```python
from build123d import *

# Parameters (mm, degrees)
ESQUISSE1_W                                       = 30
ESQUISSE1_H                                       = 44.6
BOSS_EXTRU_1_DEPTH                                = 12.2
ESQUISSE2_W                                       = 30
ESQUISSE2_H                                       = 4.3
ENL_V_MAT_EXTRU_1_DEPTH                           = 17.8
ESQUISSE3_W                                       = 30
ESQUISSE3_H                                       = 4.3
ENL_V_MAT_EXTRU_2_DEPTH                           = 22.8
FRAISAGE_POUR_VIS_T_TE_FRAIS_E_BOMB_E_D           = 5.09999996
FRAISAGE_POUR_VIS_T_TE_FRAIS_E_BOMB_E_CSINK_D     = 10.500000082
FRAISAGE_POUR_VIS_T_TE_FRAIS_E_BOMB_E_CSINK_ANGLE = 90
ESQUISSE6_W                                       = 30
ESQUISSE6_H                                       = 12.2
BOSS_EXTRU_2_DEPTH                                = 26
ESQUISSE7_W                                       = 26
ESQUISSE7_H                                       = 4.3
ENL_V_MAT_EXTRU_3_DEPTH                           = 31
FRAISAGE_POUR_VIS_T_TE_FRAIS_E_BOM_2_D            = 5.09999996
FRAISAGE_POUR_VIS_T_TE_FRAIS_E_BOM_2_CSINK_D      = 10.500000082
FRAISAGE_POUR_VIS_T_TE_FRAIS_E_BOM_2_CSINK_ANGLE  = 90


with BuildPart() as part:
    # Esquisse1 → Boss.-Extru.1 (new body)
    with BuildSketch(Plane.XY):
        with Locations((-26.085427136, 14.986432161)):
            Rectangle(ESQUISSE1_W, ESQUISSE1_H)
    extrude(amount=BOSS_EXTRU_1_DEPTH)

    # Esquisse2 → Enlèv. mat.-Extru.1 (cut)
    with BuildSketch(Plane(origin=(0, 37.286432161, 0), x_dir=(1, 0, 0), z_dir=(0, 1, 0))):
        with Locations((-26.085427136, -6.1)):
            Rectangle(ESQUISSE2_W, ESQUISSE2_H)
    extrude(amount=-ENL_V_MAT_EXTRU_1_DEPTH, mode=Mode.SUBTRACT)

    # Esquisse3 → Enlèv. mat.-Extru.2 (cut)
    with BuildSketch(Plane.XZ.offset(7.313567839)):
        with Locations((-26.085427136, 6.1)):
            Rectangle(ESQUISSE3_W, ESQUISSE3_H)
    extrude(amount=-ENL_V_MAT_EXTRU_2_DEPTH, mode=Mode.SUBTRACT)

    # Fraisage pour vis _ t_te frais_e bomb_e (through all)
    with Locations(Plane(origin=(-26.085427136, -1.313567839, 12.2), x_dir=(1, 0, 0), z_dir=(0, 0, 1))):
        with Locations((0, 0), (0, 32.6)):
            CounterSinkHole(FRAISAGE_POUR_VIS_T_TE_FRAIS_E_BOMB_E_D / 2, FRAISAGE_POUR_VIS_T_TE_FRAIS_E_BOMB_E_CSINK_D / 2, counter_sink_angle=FRAISAGE_POUR_VIS_T_TE_FRAIS_E_BOMB_E_CSINK_ANGLE)

    # Esquisse6 → Boss.-Extru.2 (add)
    with BuildSketch(Plane(origin=(0, 0, 0), x_dir=(-1, 0, 0), z_dir=(0, 0, -1))):
        with Locations((26.085427136, 13.386432161)):
            Rectangle(ESQUISSE6_W, ESQUISSE6_H)
    extrude(amount=BOSS_EXTRU_2_DEPTH)

    # Esquisse7 → Enlèv. mat.-Extru.3 (cut, through all)
    with BuildSketch(Plane.ZY.offset(41.085427136)):
        with Locations((-13, 13.386432161)):
            Rectangle(ESQUISSE7_W, ESQUISSE7_H)
    extrude(amount=-ENL_V_MAT_EXTRU_3_DEPTH, mode=Mode.SUBTRACT)

    # Fraisage pour vis _ t_te frais_e bom 2 (through all)
    with Locations(Plane(origin=(-26.085427136, 7.286432161, -13), x_dir=(-1, 0, 0), z_dir=(0, -1, 0))):
        with Locations((0, 0)):
            CounterSinkHole(FRAISAGE_POUR_VIS_T_TE_FRAIS_E_BOM_2_D / 2, FRAISAGE_POUR_VIS_T_TE_FRAIS_E_BOM_2_CSINK_D / 2, counter_sink_angle=FRAISAGE_POUR_VIS_T_TE_FRAIS_E_BOM_2_CSINK_ANGLE)


solid = part.part
```
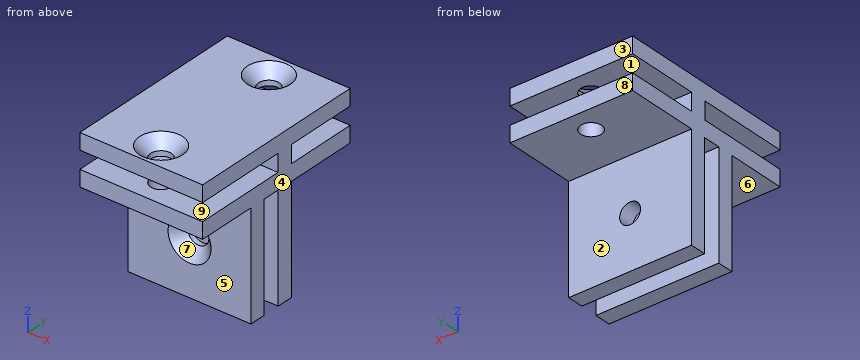
For this review, take the finished solid that the model builds, in its own axes (mm). Face numbers are marked on the shaded views. A direction names the side the tool comes from. Round coordinates to 2 decimals unless told otherwise and drop trailing zeros. Loops run counter-clockwise (first coordinate to the right, second up) from the corner with the lowest first, then second, coordinate; pieces in that order, holes last.
Q1. Insertion check: pin 1 Ø8 at (x, y) = (-26.09, 31.29) entering from +Z; pin 2 Ø5.5 at (x, y) = (-24.5, 32) entering from +Z; pin 3 Ø1.3 at (x, y) = (-29.5, 14) entering from -Z. Each pin has a flat end and moves straight along its axis. Give the tip position at first contact, or say it passes through.
Result sheet:
pin 1: stops at z = 10.96
pin 2: stops at z = 11.44
pin 3: stops at z = 0
Q2. Mouldability with a two-part tool opening along Z and no side actions: class the marked faces 6, 7, 8 and 9 as +Z half, -Z half, draft (parallel to the pull), parting line (faces both ways), or undercut.
Result sheet:
face 6: -Z half
face 7: undercut
face 8: draft
face 9: undercut
Q3. Machinability: for the marked faces 1, 2, 3, 4 and 5, which of the approach directions +Z, -Z, +X, -X, +Y, -Y give a long, thin tool a straight path to every point of the face, cutting with its end or side? Answer none if there is none.
Result sheet:
face 1: +X, -X, +Y
face 2: -Z, +X, -X, +Y
face 3: +Z, -Z, +X, -X, +Y
face 4: +Z, -Z, +X, +Y, -Y
face 5: -Z, +X, -X, -Y
Q4. Add section D-D on z = -20. Write out the cut boundary in (x, y).
Result sheet:
outline: (-41.09, 7.29) - (-11.09, 7.29) - (-11.09, 11.24) - (-41.09, 11.24) - close; (-41.09, 15.54) - (-11.09, 15.54) - (-11.09, 19.49) - (-41.09, 19.49) - close
Q5. Add section C-C on x = -38. Write out the cut boundary in (y, z), plus the area to 3 significant figures.
Result sheet:
outline: (-7.31, 0) - (7.29, 0) - (7.29, -26) - (11.24, -26) - (11.24, 0) - (15.54, 0) - (15.54, -26) - (19.49, -26) - (19.49, 0) - (37.29, 0) - (37.29, 3.95) - (19.49, 3.95) - (19.49, 8.25) - (37.29, 8.25) - (37.29, 12.2) - (-7.31, 12.2) - (-7.31, 8.25) - (15.49, 8.25) - (15.49, 3.95) - (-7.31, 3.95) - close
area: 575 mm2
Q6. Add section B-B on z = -13. Write out the cut boundary in (x, y), plus the area to 3 significant figures.
Result sheet:
outline: (-41.09, 7.29) - (-31.34, 7.29) - (-28.64, 9.99) - (-28.64, 11.24) - (-41.09, 11.24) - close; (-41.09, 15.54) - (-28.64, 15.54) - (-28.64, 19.49) - (-41.09, 19.49) - close; (-23.54, 9.99) - (-20.84, 7.29) - (-11.09, 7.29) - (-11.09, 11.24) - (-23.54, 11.24) - close; (-23.54, 15.54) - (-11.09, 15.54) - (-11.09, 19.49) - (-23.54, 19.49) - close
area: 189 mm2
Q7. Add section A-A on y = 21. Write out the cut boundary in (x, z).
Result sheet:
outline: (-41.09, 0) - (-11.09, 0) - (-11.09, 3.95) - (-41.09, 3.95) - close; (-41.09, 8.25) - (-11.09, 8.25) - (-11.09, 12.2) - (-41.09, 12.2) - close
Q8. To check wall thickness, follow line 1 along Z through (x, y) = (-21.25, 13); line 2 along X through (y, z) = (-1.5, 1.5); line 3 along Y through (x, z) = (-18.25, -9). State the ranges of each line that lie inside material, in increasing order.
Result sheet:
line 1: z = 0 to 3.95, 8.25 to 12.2
line 2: x = -41.09 to -28.63, -23.54 to -11.09
line 3: y = 7.29 to 11.24, 15.54 to 19.49
